CAD build for the part. Positions are in the model's coordinates, mm. Face numbers are marked on the shaded views. A direction names the side the tool comes from. Give positions to 0.01 mm unless a question says otherwise; leave off trailing zeros. Loops run counter-clockwise (first coordinate to the right, second up) from the corner with the lowest first, then second, coordinate; pieces in that order, holes last. Notation, with made-up numbers: M 26.5,31.5 L 60.5,31.5 A33 ccw 60.5,60.5 Z; hole C 12.5,70 d4. An arc over 180 degrees is marked long. One line per question, with ' | ' between items.
```python
from build123d import *

# Parameters (mm, degrees)
F1_DEPTH = 63.5
F2_R     = 6.35
F3_DEPTH = 63.501
F4_R     = 2.54


with BuildPart() as f1:
    # F0 (on Front) → F1 (new body)
    with BuildSketch(Plane.XZ):
        Polygon((0, 0), (-44.45, 0), (-44.45, -3.429), (-53.34, -0.193305), (-53.34, 12.506695), (-85.945848, -20.099152), (-85.945848, -25.179152), (-66.675, -44.45), (-47.625, -44.45), (-47.625, -34.925), (-38.1, -34.925), (-38.1, -44.45), (0, -44.45), align=None)
    extrude(amount=F1_DEPTH)

    # F2 (on Front) → F3 (cut, through all)
    with BuildSketch(Plane.XZ):
        with Locations((-66.895848, -22.639152)):
            Circle(F2_R)
    extrude(amount=F3_DEPTH, mode=Mode.SUBTRACT)

    # F4
    f4_edges = [f1.edges().sort_by_distance(p)[0] for p in [
        (-22.225, 0, 0),
        (0, 0, -22.225),
        (-44.45, 0, -1.7145),
        (-19.05, 0, -44.45),
        (-48.895, 0, -1.811152),
        (-38.1, 0, -39.6875),
        (-53.34, 0, 6.156695),
        (-42.8625, 0, -34.925),
        (-69.642924, 0, -3.796228),
        (-47.625, 0, -39.6875),
        (-85.945848, 0, -22.639152),
        (-57.15, 0, -44.45),
        (-76.310424, 0, -34.814576),
        (-73.245848, 0, -22.639152),
        (-85.945848, -31.75, -25.179152),
        (-66.675, -31.75, -44.45),
        (-76.310424, -63.5, -34.814576),
        (-38.1, -31.75, -44.45),
        (0, -31.75, -44.45),
        (-19.05, -63.5, -44.45),
        (-22.225, -63.5, 0),
        (0, -63.5, -22.225),
        (-44.45, -63.5, -1.7145),
        (-48.895, -63.5, -1.811152),
        (-38.1, -63.5, -39.6875),
        (-53.34, -63.5, 6.156695),
        (-42.8625, -63.5, -34.925),
        (-69.642924, -63.5, -3.796228),
        (-47.625, -63.5, -39.6875),
        (-85.945848, -63.5, -22.639152),
        (-57.15, -63.5, -44.45),
        (-73.245848, -63.5, -22.639152),
        (-47.625, -31.75, -44.45),
        (0, -31.75, 0),
        (-44.45, -31.75, 0),
        (-53.34, -31.75, 12.506695),
        (-85.945848, -31.75, -20.099152),
    ]]
    fillet(f4_edges, radius=F4_R)


solid = f1.part
```
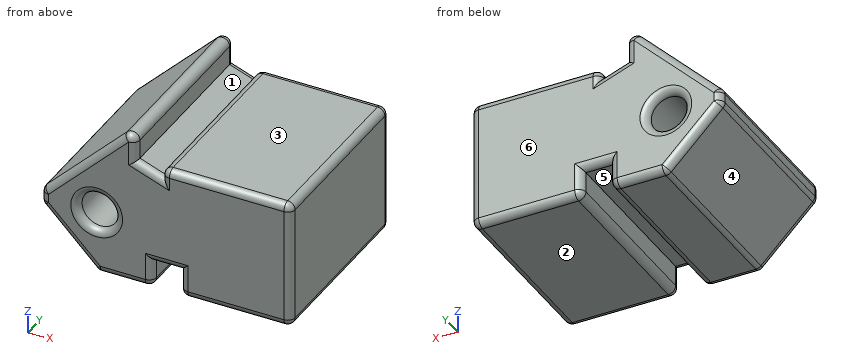
Item 1: Saw through at A-A on y = -38. Give the cut face in (x, z) (3 decimals), and give its area (3 significant figures).
Conclusion:
outline: M -85.946,-24.127 A2.54 ccw -85.202,-25.923 L -67.419,-43.706 A2.54 ccw -65.623,-44.45 L -50.165,-44.45 A2.54 ccw -47.625,-41.91 L -47.625,-34.925 L -38.1,-34.925 L -38.1,-41.91 A2.54 ccw -35.56,-44.45 L -2.54,-44.45 A2.54 ccw 0,-41.91 L 0,-2.54 A2.54 ccw -2.54,0 L -41.91,0 A2.54 ccw -44.45,-2.54 L -44.45,-3.429 L -53.34,-0.193 L -53.34,6.375 A2.54 ccw -57.676,8.171 L -85.202,-19.355 A2.54 ccw -85.946,-21.151 Z; hole C -66.896,-22.639 d12.7 | area: 3,260 mm²
Item 2: Drop flat-ended pins along their axis: P1, Ø10, axis at x = -66.9, z = -22.64, coming from the -Y side; P2, Ø5, axis at y = -8, z = -34, coming from the -X side (3 decimals); P3, Ø1.5, axis at y = -51, z = -11, coming from the -X side; P4, Ø7.5, axis at x = -43.5, y = -33, coming from the -Z side (3 decimals). Give the stop position or say it passes through.
Conclusion:
P1: through | P2: x = -79.625 | P3: x = -77.6 | P4: z = -34.925
Item 3: Saw through at B-B on x = -13.5. Give the cut face in (y, z), and give its area (3 significant figures).
Conclusion:
outline: M -63.5,-41.91 A2.54 ccw -60.96,-44.45 L -2.54,-44.45 A2.54 ccw 0,-41.91 L 0,-2.54 A2.54 ccw -2.54,0 L -60.96,0 A2.54 ccw -63.5,-2.54 Z | area: 2,820 mm²
Item 4: Mould opens along X. For the marked faces 4, 5 and 6 say: pulls with the +X half, pulls with the -X half, needs draft (parallel to the pull), parting line crosses it, or undercut.
Conclusion:
face 4: pulls with the -X half | face 5: undercut | face 6: needs draft
Item 5: 3-axis set-ups, long thin cutter, end or side, ignore diameter. For the marked faces 1, 2 and 3: which of +Z, -Z, +X, -X, +Y, -Y reach the whole face in a straight line?
Conclusion:
face 1: +Z, +Y, -Y | face 2: -Z, +X, -X, +Y, -Y | face 3: +Z, +X, +Y, -Y
Item 6: Drill centre lines: line 1 along X through (y, z) = (-46.5, -23); line 2 along Z through (x, y) = (-27.5, -10.5); line 3 along X through (y, z) = (-15.5, -18.5). Where is each one in solid material? Low to high. Write a range as [from, to].
Conclusion:
line 1: [-85.95, -73.24], [-60.56, 0] | line 2: [-44.45, 0] | line 3: [-84.35, -71.71], [-62.08, 0]
